Could you check a few things on this model? Use its own coordinates, in mm. A direction names the side the tool comes from. Give positions to 0.01 mm unless a question says otherwise; leave off trailing zeros. Loops run counter-clockwise (first coordinate to the right, second up) from the corner with the lowest first, then second, coordinate; pieces in that order, holes last.
1. Imagine slicing it at B-B (z = 0). List the corners of the cut face in (x, y) for me (3 decimals), plus the area to 3 significant figures.
2. For faces 5 (the flat face through (-9.525, -2, 14)), 6 (the flat face through (9.525, -2, 14)), 7 (the cylindrical face through (0.337, 1.565, -9.902)), 8 (the flat face through (6.477, -1, 14)), 9 (the flat face through (-8, -3.7, 11.07)), which set-ups out of +Z, -Z, +X, -X, +Y, -Y let a thin tool reach every point of the face, with its end or its side?
3. Imagine slicing it at A-A (y = -1). List the corners of the cut face in (x, z) for me (3 decimals).
4. Thinking about a two-plate mould opening in X: for faces 1 (the cylindrical face through (-8, -7.3, 14.3)), 2 (the cylindrical face through (0.736, 3.131, -19.986)), 3 (the flat face through (-6.477, -1, 14)), 4 (the flat face through (0, 3.175, 4)), which applies, +X half, -X half, draft (parallel to the pull), parting line (faces both ways), or undercut?
5. For P1, Ø5, axis at y = -3, z = 10.5, coming from the +X side (3 decimals); P2, Ø6, axis at x = 1.5, y = -4.5, coming from the +Z side (3 decimals); P3, Ø3, axis at x = 5, z = -9, coming from the -Y side; P4, Ø6, axis at y = -2.5, z = 12.5, coming from the +X side, each with a flat end and sliding along its axis, tell me the tip position at first contact or that it passes through.
6. Imagine slicing it at C-C (x = 0). List the corners of the cut face in (y, z) for me (3 decimals).
7. I need wall thicknesses on line 1 along X through (y, z) = (1.35, 0); line 2 along X through (y, z) = (-5.5, 12.5) (3 decimals); line 3 along Y through (x, z) = (4.5, 6) (3 decimals). Which ranges of each line are inside material? Lowest first, please.
```python
from build123d import *

# Parameters (mm, degrees)
SKETCH1_R               = 20.000000005
BOSS_EXTRUDE1_DEPTH     = 6.35
BOSS_EXTRUDE2_DEPTH     = 3.175
SKETCH3_R               = 1.5875
CUT_EXTRUDE1_DEPTH      = 30.525000005
CUT_EXTRUDE2_DEPTH      = 3.175
SKETCH6_W               = 9.069473667
SKETCH6_H               = 11.755238044
CUT_EXTRUDE3_DEPTH      = 14.650000005
CUT_EXTRUDE3_DEPTH_BACK = 27.350000005
CUT_EXTRUDE4_DEPTH      = 6.477
CUT_EXTRUDE4_DEPTH_BACK = 6.477


with BuildPart() as part:
    # Sketch1 → Boss-Extrude1 (new body)
    with BuildSketch(Plane(origin=(0, 0, 0), x_dir=(1, 0, 0), z_dir=(0, 1, 0))):
        Circle(SKETCH1_R)
    extrude(amount=BOSS_EXTRUDE1_DEPTH)

    # Sketch2 → Boss-Extrude2 (add)
    with BuildSketch(Plane(origin=(6.35, 0, 0), x_dir=(0, 0, -1), z_dir=(1, 0, 0))):
        with BuildLine():
            Line((-17.420082718, 0), (-17.420082718, -4.127))
            ThreePointArc((-17.420082718, -4.127), (-14.245082718, -7.302), (-11.070082718, -4.127))
            Line((-11.070082718, -4.127), (-11.070082718, -3.175))
            ThreePointArc((-11.070082718, -3.175), (-10.140146748, -0.92993597), (-7.895082718, 0))
            Line((-7.895082718, 0), (-5.849160659, 0))
            Line((-5.849160659, 0), (-5.849160659, 6.35))
            Line((-5.849160659, 6.35), (-11.070082718, 6.35))
            ThreePointArc((-11.070082718, 6.35), (-15.560210778, 4.490128061), (-17.420082718, 0))
        make_face()
    boss_extrude2 = extrude(amount=BOSS_EXTRUDE2_DEPTH)

    # Mirror1: Boss-Extrude2 across plane
    add(boss_extrude2.mirror(Plane(origin=(0, 0, 0), x_dir=(0, 0, 1), z_dir=(1, 0, 0))))

    # Sketch3 → Cut-Extrude1 (cut, through all)
    with BuildSketch(Plane(origin=(9.525, 0, 0), x_dir=(0, 0, -1), z_dir=(1, 0, 0))):
        with Locations((-14.245082718, -4.127)):
            Circle(SKETCH3_R)
    extrude(amount=-CUT_EXTRUDE1_DEPTH, mode=Mode.SUBTRACT)

    # Sketch5 → Cut-Extrude2 (cut)
    with BuildSketch(Plane.XZ):
        with BuildLine():
            Line((6.35, 18.965165441), (6.35, 7.605609073))
            ThreePointArc((6.35, 7.605609073), (0, -9.907965955), (-6.35, 7.605609073))
            Line((-6.35, 7.605609073), (-6.35, 18.965165441))
            ThreePointArc((-6.35, 18.965165441), (0, 20.000000005), (6.35, 18.965165441))
        make_face()
    extrude(amount=-CUT_EXTRUDE2_DEPTH, mode=Mode.SUBTRACT)

    # Sketch6 → Cut-Extrude3 (cut, two sides)
    with BuildSketch(Plane(origin=(6.35, 0, 0), x_dir=(0, 0, -1), z_dir=(1, 0, 0))) as cut_extrude3_sk:
        with Locations((-21.954819552, 5.877619022)):
            Rectangle(SKETCH6_W, SKETCH6_H)
    extrude(amount=CUT_EXTRUDE3_DEPTH, mode=Mode.SUBTRACT)
    extrude(cut_extrude3_sk.sketch, amount=-CUT_EXTRUDE3_DEPTH_BACK, mode=Mode.SUBTRACT)

    # Sketch7 → Cut-Extrude4 (cut, two sides)
    with BuildSketch(Plane(origin=(0, 0, 0), x_dir=(0, 0, -1), z_dir=(1, 0, 0))) as cut_extrude4_sk:
        with BuildLine():
            Line((-6.646914412, 0), (-6.646914412, 3.175))
            Line((-6.646914412, 3.175), (-7.605609073, 3.175))
            Line((-7.605609073, 3.175), (-17.420082718, 3.175))
            Line((-17.420082718, 3.175), (-17.420082718, -4.127))
            ThreePointArc((-17.420082718, -4.127), (-14.245082718, -7.302), (-11.070082718, -4.127))
            Line((-11.070082718, -4.127), (-11.070082718, -3.175))
            ThreePointArc((-11.070082718, -3.175), (-10.140146748, -0.92993597), (-7.895082718, 0))
            Line((-7.895082718, 0), (-6.646914412, 0))
        make_face()
    extrude(amount=CUT_EXTRUDE4_DEPTH, mode=Mode.SUBTRACT)
    extrude(cut_extrude4_sk.sketch, amount=-CUT_EXTRUDE4_DEPTH_BACK, mode=Mode.SUBTRACT)


solid = part.part
```
Derived:
1. outline: (-20, 0) - (-9.908, 0) - (-9.908, 3.175) - (9.908, 3.175) - (9.908, 0) - (20, 0) - (20, 6.35) - (-20, 6.35) - close
1. area: 191 mm2
2. face 5: +Z, -Z, -X, -Y
2. face 6: +Z, -Z, +X, -Y
2. face 7: -Y
2. face 8: +Z, -Y
2. face 9: -Z, +X, -X, -Y
3. outline: (-9.525, 10.208) - (-6.477, 10.208) - (-6.477, 17.42) - (-9.525, 17.42) - close; (6.477, 10.208) - (9.525, 10.208) - (9.525, 17.42) - (6.477, 17.42) - close
4. face 1: draft
4. face 2: parting line
4. face 3: undercut
4. face 4: undercut
5. P1: stops at x = 9.525
5. P2: passes through
5. P3: stops at y = 0
5. P4: stops at x = 16.81
6. outline: (0, -20) - (6.35, -20) - (6.35, 17.42) - (3.175, 17.42) - (3.175, -9.908) - (0, -9.908) - close
7. line 1: x = -20 to -9.91, 9.91 to 20
7. line 2: x = -9.525 to -6.477, 6.477 to 9.525
7. line 3: y = 3.175 to 6.35
